```python
from build123d import *

# Parameters (mm, degrees)
SKETCH1_W             = 44
SKETCH1_H             = 44
BOSS_EXTRUDE1_DEPTH   = 18
SKETCH2_R             = 15
BOSS_EXTRUDE2_DEPTH   = 6.6
M3_TAPPED_HOLE1_D     = 2.5
M3_TAPPED_HOLE1_DEPTH = 7.5
M3_TAPPED_HOLE1_TIP   = 0.751075774
SKETCH5_R             = 4
BOSS_EXTRUDE3_DEPTH   = 3.4
FILLET2_R             = 2
SKETCH6_R             = 12.784207237
CUT_EXTRUDE1_DEPTH    = 10


with BuildPart() as part:
    # Sketch1 → Boss-Extrude1 (new body)
    with BuildSketch(Plane.XY):
        Rectangle(SKETCH1_W, SKETCH1_H)
    extrude(amount=BOSS_EXTRUDE1_DEPTH)

    # Sketch2 → Boss-Extrude2 (add)
    with BuildSketch(Plane.XY.offset(18)):
        Circle(SKETCH2_R)
    extrude(amount=BOSS_EXTRUDE2_DEPTH)

    # M3 Tapped Hole1
    with Locations(Plane(origin=(0, 22, 0), x_dir=(1, 0, 0), z_dir=(0, 1, 0))):
        with Locations((-19.25, -13.5), (19.25, -13.5)):
            Hole(M3_TAPPED_HOLE1_D / 2, depth=M3_TAPPED_HOLE1_DEPTH)
            with Locations((0, 0, -(M3_TAPPED_HOLE1_DEPTH + M3_TAPPED_HOLE1_TIP / 2))):  # 118° drill point
                Cone(0, M3_TAPPED_HOLE1_D / 2, M3_TAPPED_HOLE1_TIP, mode=Mode.SUBTRACT)

    # Sketch5 → Boss-Extrude3 (add)
    with BuildSketch(Plane(origin=(0, 0, 0), x_dir=(-1, 0, 0), z_dir=(0, 0, -1))):
        with Locations((0, -13)):
            Circle(SKETCH5_R)
    extrude(amount=BOSS_EXTRUDE3_DEPTH)

    # Fillet2
    # the kernel refuses this fillet: 2 mm, written as the material it adds along each edge
    with BuildSketch(Plane(origin=(0, 0, 18), x_dir=(1, 0, 0), z_dir=(0, -1, 0))) as fillet2_piece_1:
        with BuildLine():
            CenterArc((15 + FILLET2_R, FILLET2_R), FILLET2_R, 180, 90)
            Line((15, FILLET2_R), (15, 0))
            Line((15, 0), (15 + FILLET2_R, 0))
        make_face()
    revolve(axis=Axis((0, 0, 18), (0, 0, 1)))
    # the kernel refuses this fillet: 2 mm, written as the material it takes off along each edge
    with BuildSketch(Plane(origin=(-20, 20, 16), x_dir=(0, 0, 1), z_dir=(-1, 0, 0))) as fillet2_2_piece_1_section:
        Polygon((0, 0), (FILLET2_R, 0), (FILLET2_R, FILLET2_R), (0, FILLET2_R), align=None)
    fillet2_2_piece_1 = extrude(amount=FILLET2_R, mode=Mode.PRIVATE)
    fillet2_2_piece_1 = fillet2_2_piece_1 - Plane(origin=(-20, 20, 16), x_dir=(0, -0.7071067811865475, -0.7071067811865475), z_dir=(-1, 0, 0)) * Sphere(FILLET2_R, mode=Mode.PRIVATE)
    add(fillet2_2_piece_1, mode=Mode.SUBTRACT)
    with BuildSketch(Plane(origin=(-20, -20, 16), x_dir=(-1, 0, 0), z_dir=(0, -1, 0))) as fillet2_2_piece_2_section:
        Polygon((0, 0), (FILLET2_R, 0), (FILLET2_R, -FILLET2_R), (0, -FILLET2_R), align=None)
    fillet2_2_piece_2 = extrude(amount=FILLET2_R, mode=Mode.PRIVATE)
    fillet2_2_piece_2 = fillet2_2_piece_2 - Plane(origin=(-20, -20, 16), x_dir=(0.7071067811865475, 0, -0.7071067811865475), z_dir=(0, -1, 0)) * Sphere(FILLET2_R, mode=Mode.PRIVATE)
    add(fillet2_2_piece_2, mode=Mode.SUBTRACT)
    with BuildSketch(Plane(origin=(20, -20, 16), x_dir=(1, 0, 0), z_dir=(0, -1, 0))) as fillet2_2_piece_3_section:
        Polygon((0, 0), (FILLET2_R, 0), (FILLET2_R, FILLET2_R), (0, FILLET2_R), align=None)
    fillet2_2_piece_3 = extrude(amount=FILLET2_R, mode=Mode.PRIVATE)
    fillet2_2_piece_3 = fillet2_2_piece_3 - Plane(origin=(20, -20, 16), x_dir=(-0.7071067811865475, 0, -0.7071067811865475), z_dir=(0, -1, 0)) * Sphere(FILLET2_R, mode=Mode.PRIVATE)
    add(fillet2_2_piece_3, mode=Mode.SUBTRACT)
    with BuildSketch(Plane(origin=(20, 20, 16), x_dir=(0, 0, 1), z_dir=(1, 0, 0))) as fillet2_2_piece_4_section:
        Polygon((0, 0), (FILLET2_R, 0), (FILLET2_R, -FILLET2_R), (0, -FILLET2_R), align=None)
    fillet2_2_piece_4 = extrude(amount=FILLET2_R, mode=Mode.PRIVATE)
    fillet2_2_piece_4 = fillet2_2_piece_4 - Plane(origin=(20, 20, 16), x_dir=(0, -0.7071067811865475, -0.7071067811865475), z_dir=(1, 0, 0)) * Sphere(FILLET2_R, mode=Mode.PRIVATE)
    add(fillet2_2_piece_4, mode=Mode.SUBTRACT)
    with BuildSketch(Plane(origin=(-20, -20, 2), x_dir=(-1, 0, 0), z_dir=(0, -1, 0))) as fillet2_2_piece_5_section:
        Polygon((0, 0), (FILLET2_R, 0), (FILLET2_R, FILLET2_R), (0, FILLET2_R), align=None)
    fillet2_2_piece_5 = extrude(amount=FILLET2_R, mode=Mode.PRIVATE)
    fillet2_2_piece_5 = fillet2_2_piece_5 - Plane(origin=(-20, -20, 2), x_dir=(0.7071067811865475, 0, 0.7071067811865475), z_dir=(0, -1, 0)) * Sphere(FILLET2_R, mode=Mode.PRIVATE)
    add(fillet2_2_piece_5, mode=Mode.SUBTRACT)
    with BuildSketch(Plane(origin=(20, -20, 2), x_dir=(1, 0, 0), z_dir=(0, -1, 0))) as fillet2_2_piece_6_section:
        Polygon((0, 0), (FILLET2_R, 0), (FILLET2_R, -FILLET2_R), (0, -FILLET2_R), align=None)
    fillet2_2_piece_6 = extrude(amount=FILLET2_R, mode=Mode.PRIVATE)
    fillet2_2_piece_6 = fillet2_2_piece_6 - Plane(origin=(20, -20, 2), x_dir=(-0.7071067811865475, 0, 0.7071067811865475), z_dir=(0, -1, 0)) * Sphere(FILLET2_R, mode=Mode.PRIVATE)
    add(fillet2_2_piece_6, mode=Mode.SUBTRACT)
    with BuildSketch(Plane(origin=(-20, 20, 2), x_dir=(0, 0, -1), z_dir=(-1, 0, 0))) as fillet2_2_piece_7_section:
        Polygon((0, 0), (FILLET2_R, 0), (FILLET2_R, -FILLET2_R), (0, -FILLET2_R), align=None)
    fillet2_2_piece_7 = extrude(amount=FILLET2_R, mode=Mode.PRIVATE)
    fillet2_2_piece_7 = fillet2_2_piece_7 - Plane(origin=(-20, 20, 2), x_dir=(0, -0.7071067811865475, 0.7071067811865475), z_dir=(-1, 0, 0)) * Sphere(FILLET2_R, mode=Mode.PRIVATE)
    add(fillet2_2_piece_7, mode=Mode.SUBTRACT)
    with BuildSketch(Plane(origin=(20, 20, 2), x_dir=(0, 0, -1), z_dir=(1, 0, 0))) as fillet2_2_piece_8_section:
        Polygon((0, 0), (FILLET2_R, 0), (FILLET2_R, FILLET2_R), (0, FILLET2_R), align=None)
    fillet2_2_piece_8 = extrude(amount=FILLET2_R, mode=Mode.PRIVATE)
    fillet2_2_piece_8 = fillet2_2_piece_8 - Plane(origin=(20, 20, 2), x_dir=(0, -0.7071067811865475, 0.7071067811865475), z_dir=(1, 0, 0)) * Sphere(FILLET2_R, mode=Mode.PRIVATE)
    add(fillet2_2_piece_8, mode=Mode.SUBTRACT)
    with BuildSketch(Plane(origin=(-22, 20, 18), x_dir=(0, 0, -1), z_dir=(0, -1, 0)), Plane(origin=(-20, -22, 18), x_dir=(0, 0, -1), z_dir=(1, 0, 0)), Plane(origin=(22, -20, 18), x_dir=(0, 0, -1), z_dir=(0, 1, 0)), Plane(origin=(20, 22, 0), x_dir=(0, -1, 0), z_dir=(-1, 0, 0))) as fillet2_2_piece_9:
        with BuildLine():
            CenterArc((FILLET2_R, FILLET2_R), FILLET2_R, 180, 90)
            Line((0, FILLET2_R), (0, 0))
            Line((0, 0), (FILLET2_R, 0))
        make_face()
    extrude(amount=40, mode=Mode.SUBTRACT)
    with BuildSketch(Plane(origin=(-20, -22, 0), x_dir=(0, 0, 1), z_dir=(1, 0, 0)), Plane(origin=(-22, 20, 0), x_dir=(0, 0, 1), z_dir=(0, -1, 0)), Plane(origin=(22, -20, 0), x_dir=(0, 0, 1), z_dir=(0, 1, 0)), Plane(origin=(20, 22, 18), x_dir=(0, -1, 0), z_dir=(-1, 0, 0))) as fillet2_2_piece_10:
        with BuildLine():
            CenterArc((FILLET2_R, -FILLET2_R), FILLET2_R, 90, 90)
            Line((0, -FILLET2_R), (0, 0))
            Line((0, 0), (FILLET2_R, 0))
        make_face()
    extrude(amount=40, mode=Mode.SUBTRACT)
    with BuildSketch(Plane(origin=(22, -22, 2), x_dir=(-1, 0, 0), z_dir=(0, 0, 1)), Plane(origin=(22, 22, 2), x_dir=(0, -1, 0), z_dir=(0, 0, 1))) as fillet2_2_piece_11:
        with BuildLine():
            CenterArc((FILLET2_R, -FILLET2_R), FILLET2_R, 90, 90)
            Line((0, -FILLET2_R), (0, 0))
            Line((0, 0), (FILLET2_R, 0))
        make_face()
    extrude(amount=14, mode=Mode.SUBTRACT)
    with BuildSketch(Plane(origin=(-22, -22, 2), x_dir=(1, 0, 0), z_dir=(0, 0, 1)), Plane(origin=(-22, 22, 2), x_dir=(0, -1, 0), z_dir=(0, 0, 1))) as fillet2_2_piece_12:
        with BuildLine():
            CenterArc((FILLET2_R, FILLET2_R), FILLET2_R, 180, 90)
            Line((0, FILLET2_R), (0, 0))
            Line((0, 0), (FILLET2_R, 0))
        make_face()
    extrude(amount=14, mode=Mode.SUBTRACT)

    # Sketch6 → Cut-Extrude1 (cut)
    with BuildSketch(Plane.XY.offset(24.6)):
        Circle(SKETCH6_R)
    extrude(amount=-CUT_EXTRUDE1_DEPTH, mode=Mode.SUBTRACT)


solid = part.part
```
For this review, take the finished solid that the model builds, in its own axes (mm). A direction names the side the tool comes from. Round coordinates to 2 decimals unless told otherwise and drop trailing zeros. Write each loop counter-clockwise with the first axis right and the second up, starting at its lowest first coordinate (ties: lowest second). Pieces come first, ordered by that corner, then holes.
1) Mouldability with a two-part tool opening along Y and no side actions: class faces 1 (the face through (0, 22, 9)), 2 (the face through (-21.43, -21.4, 8.9)), 3 (the face through (0, 0, 14.6)) as +Y half, -Y half, draft (parallel to the pull), parting line (faces both ways), or undercut.
Answer below:
face 1: +Y half
face 2: -Y half
face 3: undercut
2) Take a section at A-A on x = 0. Give the boundary of the cut face in (y, z), then the cut area to 3 significant figures.
Answer below:
outline: (-22, 2) arc R2 ccw to (-20, 0) - (-17, 0) - (-17, -3.4) - (-9, -3.4) - (-9, 0) - (20, 0) arc R2 ccw to (22, 2) - (22, 16) arc R2 ccw to (20, 18) - (17, 18) arc R2 cw to (15, 20) - (15, 24.6) - (12.78, 24.6) - (12.78, 14.6) - (-12.78, 14.6) - (-12.78, 24.6) - (-15, 24.6) - (-15, 20) arc R2 cw to (-17, 18) - (-20, 18) arc R2 ccw to (-22, 16) - close
area: 760 mm2
3) Take a section at C-C on z = 22.75. Give the boundary of the cut face in (x, y).
Answer below:
outline: circle Ø30 at (0, 0); hole circle Ø25.57 at (0, 0)
4) Take a section at D-D on y = 0. Give the boundary of the cut face in (x, z).
Answer below:
outline: (-22, 2) arc R2 ccw to (-20, 0) - (20, 0) arc R2 ccw to (22, 2) - (22, 16) arc R2 ccw to (20, 18) - (17, 18) arc R2 cw to (15, 20) - (15, 24.6) - (12.78, 24.6) - (12.78, 14.6) - (-12.78, 14.6) - (-12.78, 24.6) - (-15, 24.6) - (-15, 20) arc R2 cw to (-17, 18) - (-20, 18) arc R2 ccw to (-22, 16) - close
5) Insertion check: pin 1 Ø4 at (x, y) = (-15, -0.5) entering from -Z; pin 2 Ø3 at (x, y) = (6.5, -17) entering from +Z; pin 3 Ø1.5 at (x, z) = (-15.5, 1.5) entering from +Y; pin 4 Ø1.5 at (y, z) = (17.5, 18.5) entering from -X. Each pin has a flat end and moves straight along its axis. Give the tip position at first contact, or say it passes through.
Answer below:
pin 1: stops at z = 0
pin 2: stops at z = 18.02
pin 3: stops at y = 22
pin 4: stops at x = -20.97
6) Machinability: for faces 4 (the face through (0, -22, 9)), 5 (the face through (11, 7, 24.6)), 6 (the face through (-18, 0, 18)), 7 (the face through (18.06, 18.2, 13.12)), 8 (the face through (0.867, -16.905, -1.676)), which of the approach directions +Z, -Z, +X, -X, +Y, -Y give a long, thin tool a straight path to every point of the face, cutting with its end or side? Answer none if there is none.
Answer below:
face 4: +Z, -Z, +X, -X, -Y
face 5: +Z, +X, -X, +Y, -Y
face 6: +Z
face 7: +Y
face 8: -Z
7) Take a section at B-B on y = -18. Give the boundary of the cut face in (x, z), then the cut area to 3 significant figures.
Answer below:
outline: (-22, 2) arc R2 ccw to (-20, 0) - (20, 0) arc R2 ccw to (22, 2) - (22, 16) arc R2 ccw to (20, 18) - (-20, 18) arc R2 ccw to (-22, 16) - close
area: 789 mm2
8) For line 1 along X through (y, z) = (17.25, 13.5); line 2 along Z through (x, y) = (19.25, 17.5); line 3 along X through (y, z) = (6, 18.5), list the stretches that pass through material, from the lowest coordinate up.
Answer below:
line 1: x = -22 to -20.5, -18 to 18, 20.5 to 22
line 2: z = 0 to 12.25, 14.75 to 18
line 3: x = -14.48 to -11.29, 11.29 to 14.48
